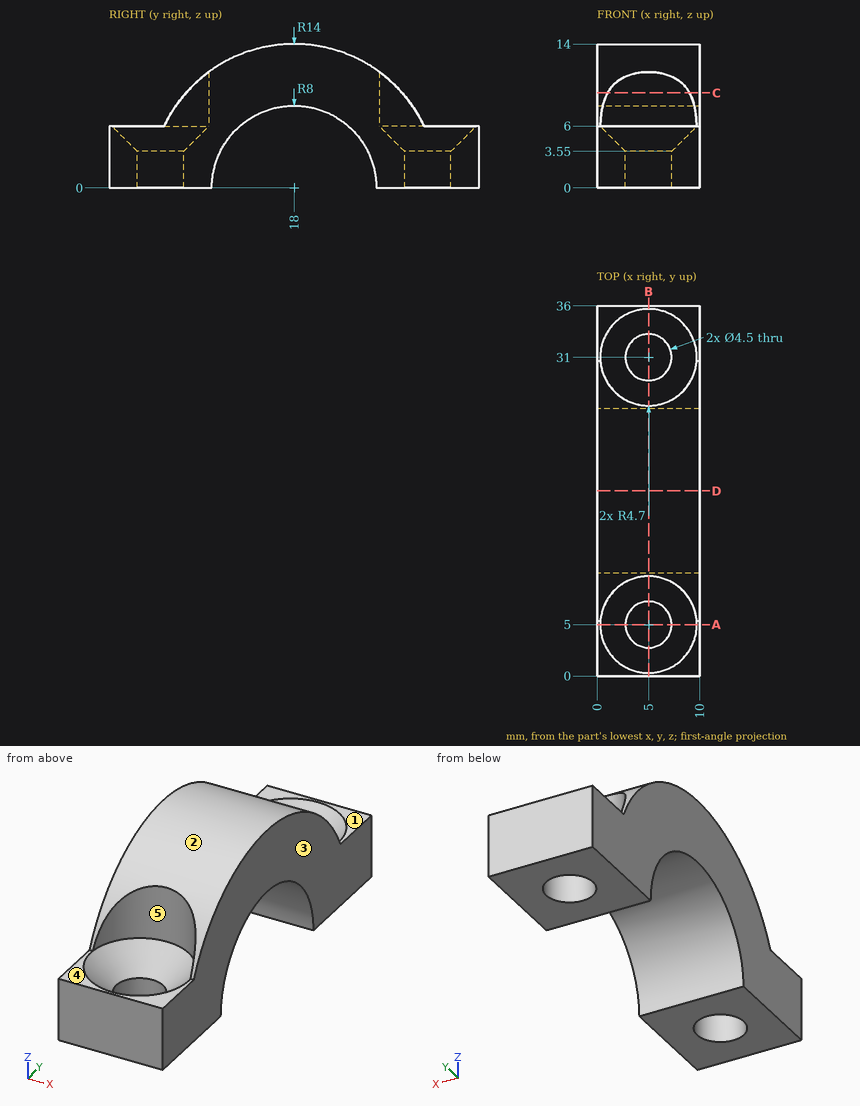
The figure shows three views and two pictorial views of one solid part (mm, origin at its lowest corner). Answer the questions. A direction names the side the tool comes from. Round coordinates to 2 decimals unless told otherwise and drop trailing zeros. Write each loop counter-clockwise with the first axis right and the second up, starting at its lowest first coordinate (ties: lowest second). Pieces come first, ordered by that corner, then holes. Notation, with made-up numbers: (18.5, -37) - (50.5, -37) arc R31 cw to (50.5, -1) - close; hole circle Ø4 at (19, 75.25). An arc over 180 degrees is marked (long way). Answer in a Markdown table with one row per item. Add a question column.
1. For the marked faces 1 and 2, determine the directions among +Z, -Z, +X, -X, +Y, -Y from which every point of the face is accessible in a straight line to the end or side of a thin tool.
2. Find the intervals of material crossed by line 1 along Y through (x, z) = (5, 1.5); line 2 along Y through (x, z) = (5, 2); line 3 along Y through (x, z) = (8.25, 7.25), in increasing order. Write a range as from..to.
3. The mould has two halves that part along X. Classify the marked faces 3, 4 and 5: +X half, -X half, draft (parallel to the pull), parting line (faces both ways), or undercut.
4. A cutting plane is placed at D-D, the plane y = 18. Determine the outline of the cut face in (x, z).
5. A cutting plane is placed at C-C, the plane z = 9.25. Determine the outline of the cut face in (x, y).
6. A cutting plane is placed at B-B, the plane x = 5. Determine the outline of the cut face in (y, z).
7. A cutting plane is placed at A-A, the plane y = 5. Determine the outline of the cut face in (x, z).
8. Given pin 1 (2 mm diameter, centred on x = 6.5, z = 12.5, fed in from -Y); pin 2 (1.5 mm diameter, centred on y = 5, z = 7.5, fed in from -X); pin 3 (6 mm diameter, centred on x = 5.5, y = 10, fed in from +Z); pin 4 (5 mm diameter, centred on x = 5, y = 5, fed in from +Z), each flat-ended and moving along its own axis, determine where each tip first touches the part or whether it passes through.
Worked out:
| question | item | result |
|---|---|---|
| 1 | face 1 | +Z, +X, -X, +Y |
| 1 | face 2 | +Z, +X, -X |
| 2 | line 1 | 0..2.75, 7.25..10.14, 25.86..28.75, 33.25..36 |
| 2 | line 2 | 0..2.75, 7.25..10.25, 25.75..28.75, 33.25..36 |
| 2 | line 3 | 8.4..14.62, 21.38..27.6 |
| 3 | face 3 | +X half |
| 3 | face 4 | draft |
| 3 | face 5 | undercut |
| 4 | outline | (0, 8) - (10, 8) - (10, 14) - (0, 14) - close |
| 5 | outline | (0, 7.49) - (1.01, 7.49) arc R4.7 cw to (8.99, 7.49) - (10, 7.49) - (10, 28.51) - (8.99, 28.51) arc R4.7 cw to (1.01, 28.51) - (0, 28.51) - close |
| 6 | outline | (0, 0) - (2.75, 0) - (2.75, 3.55) - (0.3, 6) - (0, 6) - close; (7.25, 0) - (10, 0) arc R8 cw to (26, 0) - (28.75, 0) - (28.75, 3.55) - (26.3, 6) - (26.3, 11.27) arc R14 ccw to (9.7, 11.27) - (9.7, 6) - (7.25, 3.55) - close; (33.25, 0) - (36, 0) - (36, 6) - (35.7, 6) - (33.25, 3.55) - close |
| 7 | outline | (0, 0) - (2.75, 0) - (2.75, 3.55) - (0.3, 6) - (0, 6) - close; (7.25, 0) - (10, 0) - (10, 6) - (9.7, 6) - (7.25, 3.55) - close |
| 8 | pin 1 | y = 10.02 |
| 8 | pin 2 | through |
| 8 | pin 3 | z = 13.08 |
| 8 | pin 4 | z = 3.8 |
